Verification items for the finished model (mm, model axes). Face numbers are marked on the shaded views. A direction names the side the tool comes from. Round coordinates to 2 decimals unless told otherwise and drop trailing zeros. Loops run counter-clockwise (first coordinate to the right, second up) from the corner with the lowest first, then second, coordinate; pieces in that order, holes last.
from build123d import *

# Parameters (mm, degrees)
ESQUISSE3_R             = 15
BOSS_EXTRU_2_DEPTH      = 3.6
ESQUISSE4_R             = 13.2
BOSS_EXTRU_3_DEPTH      = 12
BOSS_EXTRU_4_START      = 3.6
ESQUISSE5_R             = 13.2
BOSS_EXTRU_4_DEPTH      = 3.6
BOSS_EXTRU_5_START      = 3.6
ESQUISSE6_R             = 15
BOSS_EXTRU_5_DEPTH      = 3.6
BOSS_EXTRU_6_START      = 12
ESQUISSE7_R             = 13.2
BOSS_EXTRU_6_DEPTH      = 12
ESQUISSE8_R             = 9.6
ENL_V_MAT_EXTRU_2_DEPTH = 123


with BuildPart() as part:
    # Esquisse3 → Boss.-Extru.2 (new body)
    with BuildSketch(Plane.XY):
        Circle(ESQUISSE3_R)
    extrude(amount=-BOSS_EXTRU_2_DEPTH)

    # Esquisse4 → Boss.-Extru.3 (add)
    with BuildSketch(Plane(origin=(0, 0, -3.6), x_dir=(-1, 0, 0), z_dir=(0, 0, -1))):
        Circle(ESQUISSE4_R)
    extrude(amount=BOSS_EXTRU_3_DEPTH)

    # Esquisse5 → Boss.-Extru.4 (add)
    with BuildSketch(Plane.XY.offset(BOSS_EXTRU_4_START)):
        with Locations(Location((0, 0, 0), (0, 0, 180))):
            Circle(ESQUISSE5_R)
    extrude(amount=-BOSS_EXTRU_4_DEPTH)

    # Esquisse6 → Boss.-Extru.5 (add)
    with BuildSketch(Plane.XY.offset(3.6).offset(BOSS_EXTRU_5_START)):
        Circle(ESQUISSE6_R)
    extrude(amount=-BOSS_EXTRU_5_DEPTH)

    # Esquisse7 → Boss.-Extru.6 (add)
    with BuildSketch(Plane.XY.offset(7.2).offset(BOSS_EXTRU_6_START)):
        with Locations(Location((0, 0, 0), (0, 0, 180))):
            Circle(ESQUISSE7_R)
    extrude(amount=-BOSS_EXTRU_6_DEPTH)

    # Esquisse8 → Enlèv. mat.-Extru.2 (cut)
    with BuildSketch(Plane.XY.offset(19.2)):
        Circle(ESQUISSE8_R)
    extrude(amount=-ENL_V_MAT_EXTRU_2_DEPTH, mode=Mode.SUBTRACT)


solid = part.part
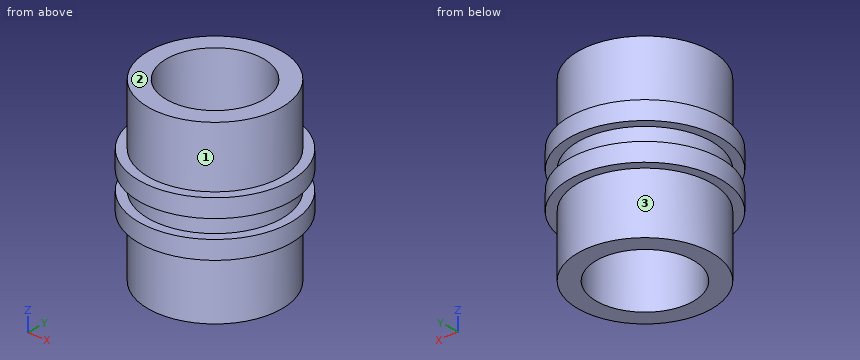
1. Scan lines: L1, parallel to Y at x = 0, z = 8; L2, parallel to Z at x = 6.5, y = -12.75; L3, parallel to Y at x = 0, z = -1. Record each from-to range of solid material in increasing order.
2. Tool access check on the marked faces 1, 2 and 3. Record the directions out of +Z, -Z, +X, -X, +Y, -Y that give a thin tool (end or side, any length) a straight path to the whole face; none if there is none.
3. Section check A-A (y = 0). Enter the section's corners in (x, z), then the cut area to 3 significant figures.
4. Section check C-C (z = -5). Enter the section's corners in (x, y), then the cut area to 3 significant figures.
5. Gauge pin test, flat ends, axial feed: P1, Ø1, axis at y = 1.5, z = 12.5, coming from the +X side; P2, Ø3, axis at x = 3.5, z = 6.5, coming from the -Y side; P3, Ø1, axis at x = -2, y = -7.5, coming from the +Z side; P4, Ø5, axis at y = 12, z = 1, coming from the +X side. Record the tip position at first contact, or that the pin passes through.
6. Section check D-D (x = 12.5). Enter the section's corners in (y, z).
Taken from the geometry:
1. L1: y = -13.2 to -9.6, 9.6 to 13.2
1. L2: z = -3.6 to 0, 3.6 to 7.2
1. L3: y = -15 to -9.6, 9.6 to 15
2. face 1: +Z
2. face 2: +Z, +X, -X, +Y, -Y
2. face 3: -Z
3. outline: (-15, -3.6) - (-13.2, -3.6) - (-13.2, -15.6) - (-9.6, -15.6) - (-9.6, 19.2) - (-13.2, 19.2) - (-13.2, 7.2) - (-15, 7.2) - (-15, 3.6) - (-13.2, 3.6) - (-13.2, 0) - (-15, 0) - close; (9.6, -15.6) - (13.2, -15.6) - (13.2, -3.6) - (15, -3.6) - (15, 0) - (13.2, 0) - (13.2, 3.6) - (15, 3.6) - (15, 7.2) - (13.2, 7.2) - (13.2, 19.2) - (9.6, 19.2) - close
3. area: 276 mm2
4. outline: circle Ø26.4 at (0, 0); hole circle Ø19.2 at (0, 0)
4. area: 258 mm2
5. P1: stops at x = 13.16
5. P2: stops at y = -14.87
5. P3: passes through
5. P4: stops at x = 11.43
6. outline: (-8.29, -3.6) - (-4.24, -3.6) - (-4.24, -15.6) - (4.24, -15.6) - (4.24, -3.6) - (8.29, -3.6) - (8.29, 0) - (4.24, 0) - (4.24, 3.6) - (8.29, 3.6) - (8.29, 7.2) - (4.24, 7.2) - (4.24, 19.2) - (-4.24, 19.2) - (-4.24, 7.2) - (-8.29, 7.2) - (-8.29, 3.6) - (-4.24, 3.6) - (-4.24, 0) - (-8.29, 0) - close
